Source: CAD feature listing. Evaluate the final solid. Frame: model axes, mm. Give positions to 0.01 mm unless a question says otherwise; leave off trailing zeros. Order: outer loops, then holes, each group sorted by start corner. A loop starts at its lowest first (then second) coordinate and runs counter-clockwise, first axis right, second up. Notation, with made-up numbers: M 47.25,78 L 66.25,78 A13 ccw 66.25,88 Z; hole C 74,40 d8. An arc over 180 degrees is marked long. Use CSV: the item, a comma, the result in double quotes. Start each with the question number.
Item 1: Section query C-C on y = -14. Return loops of the section in (x, z) (3 decimals).
Item 2: Section query D-D on x = -41.91. Return loops of the section in (y, z) (3 decimals), and give its area (3 significant figures).
Item 3: Pull-direction query (X, two-part tool) for faces 1 (the face through (-18.72, -12.34, -35.57)), 2 (the face through (-1, -12, 50.8)), 3 (the face through (63.5, -12, -1)); classes: +X half, -X half, draft (parallel to the pull), parting line (faces both ways), or undercut.
Item 4: Section query B-B on z = -38.1. Return loops of the section in (x, y), and give its area (3 significant figures).
Item 5: Ray query, probe 1 along X at (y, z) = (-24, 38); probe 2 along Z at (x, y) = (-41.91, -19) (3 decimals); probe 3 along Z at (x, y) = (-19.05, -25). Return the intervals inside material, ascending. Write a range as from..to.
Item 6: First-contact query: pin 1 (3 mm diameter, centred on x = 31.75, z = -38.1, fed in from -Y). Flat tip, straight axial feed; report the tip coordinate or a pass-through.
Item 7: Section query A-A on z = 29.21. Return loops of the section in (x, y) (3 decimals), and give its area (3 significant figures).
from build123d import *

# Parameters (mm, degrees)
F0_W     = 127
F0_H     = 101.6
F1_DEPTH = 12.7
F2_DEPTH = 25.4
F3_R     = 9.525
F4_DEPTH = 50.801
F6_D     = 5.1054


with BuildPart() as f1:
    # F0 (on Front) → F1 (new body, symmetric)
    with BuildSketch(Plane.XZ):
        Rectangle(F0_W, F0_H)
    extrude(amount=F1_DEPTH, both=True)

    # F2 (add): a face of the model
    f2_faces = [f1.faces().sort_by_distance(p)[0] for p in [
        (0, -12.7, 0),
    ]]
    extrude(f2_faces, amount=F2_DEPTH)

    # F3 (on face) → F4 (cut, through all)
    with BuildSketch(Plane.XZ.offset(38.1)):
        with Locations((-41.91, 29.21)):
            Circle(F3_R)
    extrude(amount=-F4_DEPTH, mode=Mode.SUBTRACT)

    # F6 (through all)
    with Locations(Plane.XZ.offset(38.1)):
        with Locations((31.75, 38.1), (31.75, -38.1), (-19.05, -38.1)):
            Hole(F6_D / 2)


solid = f1.part
Verdict:
1,outline,"M -63.5,-50.8 L 63.5,-50.8 L 63.5,50.8 L -63.5,50.8 Z; hole C -41.91,29.21 d19.05; hole C -19.05,-38.1 d5.105; hole C 31.75,-38.1 d5.105; hole C 31.75,38.1 d5.105"
2,outline,"M -38.1,-50.8 L 12.7,-50.8 L 12.7,19.685 L -38.1,19.685 Z; M -38.1,38.735 L 12.7,38.735 L 12.7,50.8 L -38.1,50.8 Z"
2,area,"4,190 mm2"
3,face 1,"undercut"
3,face 2,"draft"
3,face 3,"+X half"
4,outline,"M -63.5,-38.1 L -21.6,-38.1 L -21.6,12.7 L -63.5,12.7 Z; M -16.5,-38.1 L 29.2,-38.1 L 29.2,12.7 L -16.5,12.7 Z; M 34.3,-38.1 L 63.5,-38.1 L 63.5,12.7 L 34.3,12.7 Z"
4,area,"5,930 mm2"
5,probe 1,"-63.5..-45.58, -38.24..29.2, 34.3..63.5"
5,probe 2,"-50.8..19.685, 38.735..50.8"
5,probe 3,"-50.8..-40.65, -35.55..50.8"
6,pin 1,"through"
7,outline,"M -63.5,-38.1 L -51.435,-38.1 L -51.435,12.7 L -63.5,12.7 Z; M -32.385,-38.1 L 63.5,-38.1 L 63.5,12.7 L -32.385,12.7 Z"
7,area,"5,480 mm2"
